Autodesk Inventor part; units mm, degrees
ref_plane "YZ Plane" through (0, 0, 0) normal (1, 0, 0) x (0, 1, 0)
ref_plane "XZ Plane" through (0, 0, 0) normal (0, 1, 0) x (-1, 0, 0)
ref_plane "XY Plane" through (0, 0, 0) normal (0, 0, 1) x (1, 0, 0)
sketch "Szkic1" plane through (0, 0, 0) normal (0, 1, 0) x (-1, 0, 0)
  line L0 (8.89, -1.91) -> (8.89, -57.14)
  line L1 (6.98, -59.05) -> (1.91, -59.05)
  line L2 (0, -57.14) -> (0, -1.91)
  line L3 (6.98, 0) -> (8.89, -1.91)
  line L4 (1.91, 0) -> (0, -1.91)
  line L5 (0, -57.14) -> (1.91, -59.05)
  line L6 (6.98, -59.05) -> (8.89, -57.14)
  line L7 (6.98, 0) -> (1.91, 0)
  line L8 (4.445, -59.05) -> (4.445, 0)
  circle A0 centre (4.445, -6.35) radius 0.75
  circle A1 centre (4.445, -21.59) radius 0.75
  circle A2 centre (4.445, -36.83) radius 0.75
  circle A3 centre (4.445, -52.07) radius 0.75
  line L9 (7.89, -56.7258) -> (6.5658, -58.05)
  line L10 (6.5658, -58.05) -> (2.3242, -58.05)
  line L11 (2.3242, -58.05) -> (1, -56.7258)
  line L12 (1, -56.7258) -> (1, -2.3242)
  line L13 (1, -2.3242) -> (2.3242, -1)
  line L14 (2.3242, -1) -> (6.5658, -1)
  line L15 (6.5658, -1) -> (7.89, -2.3242)
  line L16 (7.89, -2.3242) -> (7.89, -56.7258)
  point P0 (0, 0)
  point P1 (8.89, -59.05)
  point P2 (8.89, 0)
  point P3 (0, -59.05)
  dimension "d0" = 8.89
  dimension "d2" = 1.91
  dimension "d3" = 1.91
  dimension "d4" = 1.91
  dimension "d5" = 1.91
  dimension "d6" = 1.91
  dimension "d7" = 1.91
  dimension "d8" = 1.91
  dimension "d9" = 1.91
  dimension "d10" = 1.5
  dimension "d11" = 6.35
  dimension "d14" = 15.24
  dimension "d19" = 1
extrude "Wyciągnięcie proste1" add sketch "Szkic1" along normal blind 1 contours L14 L15 L16 L9 L10 L8 A3 A2 A1 A0 | L8 A0 A1 A2 A3 L10 L11 L12 L13 L14
properties part number "vin"
Input: part model. Units: mm. Frame: model coordinates. Coordinates: 2 decimals unless noted, no trailing zeros. Loops run counter-clockwise (first coordinate to the right, second up) from the corner with the lowest first, then second, coordinate; pieces in that order, holes last.
Q1. Mould query, pull axis X, two halves, no side actions, for faces 1 (the flat face through (-4.4, 0.5, -1)), 2 (the cylindrical face through (-4.28, 0.49, -20.86)), 3 (the cylindrical face through (-4.347, 0.493, -52.814)), 4 (the flat face through (-7.89, 0.5, -29.1)). Classes: +X half, -X half, draft (parallel to the pull), parting line (faces both ways), or undercut.
Results are:
face 1: draft
face 2: undercut
face 3: undercut
face 4: -X half
Q2. Section B-B, the plane z = -6.35. Return the cut outline in (x, y) (3 decimals), and give its area (3 significant figures).
Results are:
outline: (-7.89, 0) - (-5.195, 0) - (-5.195, 1) - (-7.89, 1) - close; (-3.695, 0) - (-1, 0) - (-1, 1) - (-3.695, 1) - close
area: 5.39 mm2
Q3. Line query: line 1 along Z through (x, y) = (-4.5, 0.15); line 2 along Z through (x, y) = (-4.75, 0.85); line 3 along X through (y, z) = (0.5, -21.59) (3 decimals). Output: solid intervals per line, ascending.
Results are:
line 1: z = -58.05 to -52.82, -51.32 to -37.58, -36.08 to -22.34, -20.84 to -7.1, -5.6 to -1
line 2: z = -58.05 to -52.76, -51.38 to -37.52, -36.14 to -22.28, -20.9 to -7.04, -5.66 to -1
line 3: x = -7.89 to -5.195, -3.695 to -1
Q4. Section A-A, the plane y = 0.5. Return the cut outline in (x, z) (3 decimals).
Results are:
outline: (-7.89, -56.726) - (-6.566, -58.05) - (-2.324, -58.05) - (-1, -56.726) - (-1, -2.324) - (-2.324, -1) - (-6.566, -1) - (-7.89, -2.324) - close; hole circle Ø1.5 at (-4.445, -52.07); hole circle Ø1.5 at (-4.445, -36.83); hole circle Ø1.5 at (-4.445, -21.59); hole circle Ø1.5 at (-4.445, -6.35)
